Verification items for the finished model (mm, model axes). Face numbers are marked on the shaded views. Round coordinates to 2 decimals unless told otherwise and drop trailing zeros. Loops run counter-clockwise (first coordinate to the right, second up) from the corner with the lowest first, then second, coordinate; pieces in that order, holes last. Notation, with made-up numbers: (-34.75, 30) -> (3.25, 30) arc R14 cw to (3.25, 38) -> close; hole circle Ø3 at (47.25, 32.5). An arc over 180 degrees is marked (long way). Use a Markdown table: item, result. Add a question column.
```python
from build123d import *

# Parameters (mm, degrees)
SKETCH5_W           = 200
SKETCH5_H           = 200
BOSS_EXTRUDE2_DEPTH = 200
SHELL2_T            = -20
SKETCH6_R           = 26
CUT_EXTRUDE2_DEPTH  = 51.6


with BuildPart() as part:
    # Sketch5 → Boss-Extrude2 (new body)
    with BuildSketch(Plane.XY):
        Rectangle(SKETCH5_W, SKETCH5_H)
    extrude(amount=BOSS_EXTRUDE2_DEPTH)

    # Shell2
    shell2_openings = [part.faces().sort_by_distance(p)[0] for p in [
        (0, 0, 0),
    ]]
    offset(amount=SHELL2_T, openings=shell2_openings, kind=Kind.INTERSECTION)

    # Sketch6 → Cut-Extrude2 (cut)
    with BuildSketch(Plane.XY.offset(200)):
        Circle(SKETCH6_R)
    extrude(amount=-CUT_EXTRUDE2_DEPTH, mode=Mode.SUBTRACT)


solid = part.part
```
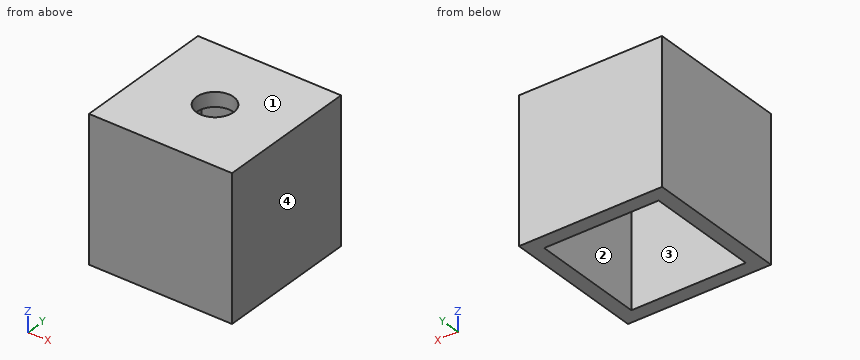
1) Sectioned sample at C-C on z = 73.5. Enter the section's corners in (x, y).
2) Sectioned sample at A-A on x = 0. Enter the section's corners in (y, z), then the cut area to 3 significant figures.
3) Sectioned sample at D-D on y = 58. Enter the section's corners in (x, z), then the cut area to 3 significant figures.
4) Thickness scan on line 1 (X direction, y = 34.5, z = 161.5); line 2 (Y direction, x = 0, z = 187.5). Record the ranges inside material, lowest first.
5) Go/stop test with a flat-tipped pin: pin 1 (1.5 mm diameter, centred on x = 62.5, y = 59.5, fed in from -Z). Record where the tip stops, or that it passes through.
6) Release check for a two-part mould opening along X. For the marked faces 1, 2, 3 and 4 record: released by +X, released by -X, zero draft, split by the parting line, or undercut.
Geometry results:
| question | item | result |
|---|---|---|
| 1 | outline | (-100, -100) -> (100, -100) -> (100, 100) -> (-100, 100) -> close; hole (-80, -80) -> (80, -80) -> (80, 80) -> (-80, 80) -> close |
| 2 | outline | (-100, 0) -> (-80, 0) -> (-80, 180) -> (-26, 180) -> (-26, 200) -> (-100, 200) -> close; (26, 180) -> (80, 180) -> (80, 0) -> (100, 0) -> (100, 200) -> (26, 200) -> close |
| 2 | area | 10,200 mm^2 |
| 3 | outline | (-100, 0) -> (-80, 0) -> (-80, 180) -> (80, 180) -> (80, 0) -> (100, 0) -> (100, 200) -> (-100, 200) -> close |
| 3 | area | 11,200 mm^2 |
| 4 | line 1 | -100 to -80, 80 to 100 |
| 4 | line 2 | -100 to -26, 26 to 100 |
| 5 | pin 1 | z = 180 |
| 6 | face 1 | zero draft |
| 6 | face 2 | undercut |
| 6 | face 3 | undercut |
| 6 | face 4 | released by +X |
